Geometry: final body of the model. Coordinates: model frame, mm. A direction names the side the tool comes from. Round coordinates to 2 decimals unless told otherwise and drop trailing zeros. Order: outer loops, then holes, each group sorted by start corner. A loop starts at its lowest first (then second) coordinate and runs counter-clockwise, first axis right, second up. Notation, with made-up numbers: (-20.75, 29.5) - (-3.75, 29.5) arc R20 ccw to (-3.75, 46.5) - close; hole circle Ø9 at (10, 20). An arc over 180 degrees is marked (long way). Put each result on its own line as item: value. Start each with the question number.
(1) Pull-direction query (Z, two-part tool) for faces 6 (the face through (12.5, 11, 2)), 7 (the face through (18, 11, 4)), 8 (the face through (20.5, 11.2, 8)); classes: released by +Z, released by -Z, zero draft, split by the parting line, or undercut.
(2) Section C-C (y = 14.5). Output: boundary loops of the cut face in (x, z).
(3) Access query for faces 1 (the face through (20.5, 0.75, 11.3)), 2 (the face through (21, 8, 20)), 3 (the face through (20.5, 3.75, 13.6)), 4 (the face through (-2, 12, 0)), 5 (the face through (6, 22.7, 2)). Directions: +Z, -Z, +X, -X, +Y, -Y. A direction counts if a zero-diameter tool reaches every point of the face in a straight line with its end or side. Return the directions, or none.
(4) Section D-D (z = 22.5). Output: boundary loops of the cut face in (x, y), and give its area (3 significant figures).
(5) Pin query (flat end, axial travel): P1, Ø0.8, axis at x = 20.5, z = 12, coming from the -Y side; P2, Ø4.5, axis at y = 8.5, z = 2.5, coming from the +X side; P3, Ø1.1, axis at x = -8, y = 13, coming from the +Z side. Return the tip coordinate at first contact, or that it passes through.
(6) Section B-B (z = 14.25). Output: boundary loops of the cut face in (x, y), and give its area (3 significant figures).
(7) Material intervals for L1, parallel to X at y = 17.25, z = 6.25; L2, parallel to X at y = 4.25, z = 3.5; L3, parallel to X at y = -0.5, z = 2, sorted ascending. Write a range as [from, to].
(8) Section A-A (x = 8). Output: boundary loops of the cut face in (y, z), and give its area (3 significant figures).
from build123d import *

# Parameters (mm, degrees)
SKETCH_1_W          = 18.5
SKETCH_1_H          = 28.7
SKETCH_1_W_2        = 12.5
SKETCH_1_H_2        = 22.7
EXTRUDE_1_DEPTH     = 5
EXTRUDE_2_DEPTH     = 28.7
CHAMFER_1_SIZE      = 1
SKETCH_3_W          = 13.25
SKETCH_3_H          = 3.75
CUT_EXTRUDE_1_DEPTH = 47.975951294
FILLET_1_R          = 1
CUT_EXTRUDE_2_DEPTH = 47.838045433
FILLET_2_R          = 1
SKETCH_6_R          = 2.25
CUT_EXTRUDE_3_DEPTH = 47.838045433


with BuildPart() as part:
    # 草图1 → 凸台-拉伸1 (new body)
    with BuildSketch(Plane.XY):
        with Locations((6.25, 11.35)):
            Rectangle(SKETCH_1_W, SKETCH_1_H)
        with Locations((6.25, 11.35)):
            Rectangle(SKETCH_1_W_2, SKETCH_1_H_2, mode=Mode.SUBTRACT)
    extrude(amount=EXTRUDE_1_DEPTH)

    # 草图2 → 凸台-拉伸2 (add)
    with BuildSketch(Plane.XZ.offset(3)):
        Polygon((-3, 5), (-3, 4), (-8.5, 4), (-8.5, 26), (-7.5, 26), (-7.5, 5), align=None)
        Polygon((20, 26), (20, 5), (15.5, 5), (15.5, 4), (21, 4), (21, 26), align=None)
    extrude(amount=-EXTRUDE_2_DEPTH)

    # 倒角1
    chamfer_1_edges = [part.edges().sort_by_distance(p)[0] for p in [
        (-8.5, 11.35, 4),
        (21, 11.35, 4),
    ]]
    chamfer(chamfer_1_edges, length=CHAMFER_1_SIZE)

    # 草图3 → 切除-拉伸1 (cut, through all)
    with BuildSketch(Plane(origin=(21, 0, 0), x_dir=(0, 0, -1), z_dir=(1, 0, 0))):
        with BuildLine():
            ThreePointArc((-25.75, 0.75), (-25.700415908, 1.357801045), (-25.552974874, 1.949528884))
            Line((-25.552974874, 1.949528884), (-24.074717326, 10.949460339))
            Line((-24.074717326, 10.949460339), (-5, 25.7))
            Line((-5, 25.7), (-26, 25.7))
            Line((-26, 25.7), (-26, 0.75))
            Line((-26, 0.75), (-25.75, 0.75))
        make_face()
        with BuildLine():
            Line((-26, -3), (-22, -3))
            ThreePointArc((-22, -3), (-24.651650429, -1.901650429), (-25.75, 0.75))
            Line((-25.75, 0.75), (-26, 0.75))
            Line((-26, 0.75), (-26, -3))
        make_face()
        with BuildLine():
            Line((-22, -3), (-18.25, -3))
            Line((-18.25, -3), (-18.25, 0.75))
            ThreePointArc((-18.25, 0.75), (-19.348349571, -1.901650429), (-22, -3))
        make_face()
        with Locations((-11.625, -1.125)):
            Rectangle(SKETCH_3_W, SKETCH_3_H)
    extrude(amount=-CUT_EXTRUDE_1_DEPTH, mode=Mode.SUBTRACT)

    # 圆角1
    fillet_1_edges = [part.edges().sort_by_distance(p)[0] for p in [
        (-8, 0.75, 18.25),
        (20.5, 0.75, 18.25),
    ]]
    fillet(fillet_1_edges, radius=FILLET_1_R)

    # 草图5 → 切除-拉伸2 (cut, through all)
    with BuildSketch(Plane(origin=(21, 0, 0), x_dir=(0, 0, -1), z_dir=(1, 0, 0))):
        Polygon((-19.428547646, 3.75), (-19.428547646, 10.75), (-8, 19.587732294), (-8, 3.75), align=None)
    extrude(amount=-CUT_EXTRUDE_2_DEPTH, mode=Mode.SUBTRACT)

    # 圆角2
    fillet_2_edges = [part.edges().sort_by_distance(p)[0] for p in [
        (-8, 3.75, 8),
        (-8, 3.75, 19.428547646),
        (-8, 10.75, 19.428547646),
        (-8, 19.587732294, 8),
        (20.5, 3.75, 8),
        (20.5, 3.75, 19.428547646),
        (20.5, 10.75, 19.428547646),
        (20.5, 19.587732294, 8),
    ]]
    fillet(fillet_2_edges, radius=FILLET_2_R)

    # 草图6 → 切除-拉伸3 (cut, through all)
    with BuildSketch(Plane(origin=(21, 0, 0), x_dir=(0, 0, -1), z_dir=(1, 0, 0))):
        with Locations((-22, 0.75)):
            Circle(SKETCH_6_R)
    extrude(amount=-CUT_EXTRUDE_3_DEPTH, mode=Mode.SUBTRACT)


solid = part.part
Checks:
1. face 6: zero draft
1. face 7: released by -Z
1. face 8: undercut
2. outline: (-8.5, 5) - (-7.5, 4) - (-3, 4) - (-3, 0) - (0, 0) - (0, 5) - (-7.5, 5) - (-7.5, 8) - (-8.5, 8) - close; (-8.5, 14.58) - (-7.5, 14.58) - (-7.5, 19.48) - (-8.5, 19.48) - close; (12.5, 0) - (15.5, 0) - (15.5, 4) - (20, 4) - (21, 5) - (21, 8) - (20, 8) - (20, 5) - (12.5, 5) - close; (20, 14.58) - (21, 14.58) - (21, 19.48) - (20, 19.48) - close
3. face 1: +X, -X, -Y
3. face 2: +Z, -Z, +X, +Y, -Y
3. face 3: +X, -X
3. face 4: -Z, +X, -X, +Y, -Y
3. face 5: +Z, -Z
4. outline: (-8.5, -2.97) - (-7.5, -2.97) - (-7.5, -1.44) - (-8.5, -1.44) - close; (-8.5, 2.94) - (-7.5, 2.94) - (-7.5, 12.17) - (-8.5, 12.17) - close; (20, -2.97) - (21, -2.97) - (21, -1.44) - (20, -1.44) - close; (20, 2.94) - (21, 2.94) - (21, 12.17) - (20, 12.17) - close
4. area: 21.5 mm²
5. P1: stops at y = 0.75
5. P2: stops at x = 20.75
5. P3: stops at z = 22.13
6. outline: (-8.5, 0.75) - (-7.5, 0.75) - (-7.5, 3.75) - (-8.5, 3.75) - close; (-8.5, 14.75) - (-7.5, 14.75) - (-7.5, 18.55) - (-8.5, 18.55) - close; (20, 0.75) - (21, 0.75) - (21, 3.75) - (20, 3.75) - close; (20, 14.75) - (21, 14.75) - (21, 18.55) - (20, 18.55) - close
6. area: 13.6 mm²
7. L1: x = [-8.5, -7.5], [20, 21]
7. L2: x = [-3, 0], [12.5, 15.5]
7. L3: x = [-3, 15.5]
8. outline: (-3, 0) - (0, 0) - (0, 5) - (-3, 5) - close; (22.7, 0) - (25.7, 0) - (25.7, 5) - (22.7, 5) - close
8. area: 30.0 mm²
